Autodesk Inventor part; units mm, degrees
ref_plane "YZ Plane" through (0, 0, 0) normal (1, 0, 0) x (0, 1, 0)
ref_plane "XZ Plane" through (0, 0, 0) normal (0, 1, 0) x (-1, 0, 0)
ref_plane "XY Plane" through (0, 0, 0) normal (0, 0, 1) x (1, 0, 0)
sketch "Sketch1" plane through (0, 0, 0) normal (0, 1, 0) x (-1, 0, 0)
  circle A0 centre (0, 0) radius 39.5
  circle A1 centre (0, 0) radius 40.5
  dimension "d0" = 79
  dimension "d1" = 81
extrude "Extrusion1" add sketch "Sketch1" along normal blind 2
sketch "Sketch21" plane through (0, 2, 0) normal (0, 1, 0) x (1, 0, 0)
  line L0 (-40.5, -40.5) -> (40.5, -40.5)
  line L1 (40.5, -40.5) -> (40.5, 40.5)
  line L2 (40.5, 40.5) -> (-40.5, 40.5)
  line L3 (-40.5, 40.5) -> (-40.5, -40.5)
  line L4 (-40.5, -40.5) -> (40.5, 40.5) construction
  line L5 (40.5, -40.5) -> (-40.5, 40.5) construction
  circle A0 centre (0, 0) radius 40.5
  dimension "d111" = 81
  dimension "d112" = 81
extrude "Extrusion21" add sketch "Sketch21" against normal blind 2 contours L3 A0 L0 | A0 L1 L0 | L3 L2 A0 | A0 L2 L1
fillet "Fillet3" radius 20 4 edges at (-40.5, 1, -40.5) (40.5, 1, -40.5) (40.5, 1, 40.5) (-40.5, 1, 40.5)
sketch "Sketch24" plane through (0, 0, 0) normal (0, -1, 0) x (1, 0, 0)
  arc A0 (-20.5, 40.5) -> (-40.5, 20.5) centre (-20.5, 20.5) ccw
  circle A1 centre (0, 0) radius 39.5
  arc A2 (-20.5, 40.5) -> (-40.5, 20.5) centre (-20.5, 20.5) ccw
  line L0 (-40.5, 20.5) -> (-40.5, -20.5)
  arc A3 (-40.5, -20.5) -> (-20.5, -40.5) centre (-20.5, -20.5) ccw
  line L1 (-20.5, -40.5) -> (20.5, -40.5)
  arc A4 (20.5, -40.5) -> (40.5, -20.5) centre (20.5, -20.5) ccw
  line L2 (40.5, -20.5) -> (40.5, 20.5)
  arc A5 (40.5, 20.5) -> (20.5, 40.5) centre (20.5, 20.5) ccw
  line L3 (20.5, 40.5) -> (-20.5, 40.5)
  line L4 (-20, -40) -> (20, -40)
  line L5 (40, -20) -> (40, 20)
  line L6 (20, 40) -> (-20, 40)
  line L7 (-40, 20) -> (-40, -20)
  line L8 (-40, -40) -> (40, 40) construction
  line L9 (40, -40) -> (-40, 40) construction
  arc A6 (-38, 40) -> (-40, 38) centre (-38, 38) ccw
  arc A7 (40, 20) -> (20, 40) centre (20, 20) ccw
  arc A8 (-20, 40) -> (-40, 20) centre (-20, 20) ccw
  arc A9 (-40, -20) -> (-20, -40) centre (-20, -20) ccw
  arc A10 (20, -40) -> (40, -20) centre (20, -20) ccw
  dimension "d133" = 80
  dimension "d134" = 80
  dimension "d135" = 2
  dimension "d136" = 20
extrude "Extrusion24" add sketch "Sketch24" along normal blind 40 contours L3 A5 L2 A4 L1 A3 L0 A0
sketch "Sketch25" plane through (0, 0, 0) normal (0, -1, 0) x (1, 0, 0)
  circle A0 centre (-31, -31) radius 2
  line L0 (0, 0) -> (-40.0942, -40.0942)
  line L1 (0, 0) -> (0, -34.7078)
  circle A1 centre (31, -31) radius 2
  circle A2 centre (31, 31) radius 2
  circle A3 centre (-31, 31) radius 2
  dimension "d139" = 4
  dimension "d140" = 31
  dimension "d141" = 45
  dimension "d144" = 360
extrude "Extrusion25" cut sketch "Sketch25" against normal blind 10
properties part number "Motor mount (plain)"
Input: part model. Units: mm. Frame: model coordinates. A direction names the side the tool comes from. Give positions to 0.01 mm unless a question says otherwise; leave off trailing zeros. Order: outer loops, then holes, each group sorted by start corner. A loop starts at its lowest first (then second) coordinate and runs counter-clockwise, first axis right, second up. Notation, with made-up numbers: M 22.5,54 L 48.5,54 A26 cw 48.5,87 Z; hole C -24.5,-33.5 d1. An arc over 180 degrees is marked long. Return JSON: item names as keys, results as strings.
Item 1: Cut plane D-D (z = 31). Return loops of the section in (x, y), then the cut area to 3 significant figures.
Solutions:
{"outline": "M -37.52,-40 L -36.7,-40 L -36.7,0 L -33,0 L -33,2 L -37.52,2 Z; M -29,0 L -24.48,0 L -24.48,2 L -29,2 Z; M 24.48,0 L 29,0 L 29,2 L 24.48,2 Z; M 33,0 L 36.7,0 L 36.7,-40 L 37.52,-40 L 37.52,2 L 33,2 Z", "area": "102 mm^2"}
Item 2: Access query for faces 1 (the cylindrical face through (33.986, -19.72, 34.297)), 2 (the flat face through (0, -19, -40.5)). Directions: +Z, -Z, +X, -X, +Y, -Y. A direction counts if a zero-diameter tool reaches every point of the face in a straight line with its end or side. Return the directions, or none.
Solutions:
{"face 1": "-Y", "face 2": "-Z, +X, -X, +Y, -Y"}
Item 3: Ray query, probe 1 along Z at (x, y) = (-17.5, -27.5); probe 2 along Z at (x, y) = (31, 1). Return the intervals inside material, ascending.
Solutions:
{"probe 1": "-40.5 to -40, 40 to 40.5", "probe 2": "-37.52 to -33, -29 to -24.48, 24.48 to 29, 33 to 37.52"}
Item 4: First-contact query: P1, Ø8, axis at x = 18.5, z = -29.5, coming from the +Y side; P2, Ø5, axis at x = 31, z = 31, coming from the -Y side. Flat tips, straight axial feed; report the tip coordinate or a pass-through.
Solutions:
{"P1": "through", "P2": "y = 0"}
Item 5: Cut plane C-C (y = -14). Return loops of the section in (x, z).
Solutions:
{"outline": "M -40.5,-20.5 A20 ccw -20.5,-40.5 L 20.5,-40.5 A20 ccw 40.5,-20.5 L 40.5,20.5 A20 ccw 20.5,40.5 L -20.5,40.5 A20 ccw -40.5,20.5 Z; hole M -40,-20 A20 ccw -20,-40 L 20,-40 A20 ccw 40,-20 L 40,20 A20 ccw 20,40 L -20,40 A20 ccw -40,20 Z"}
Item 6: Cut plane B-B (z = 0). Return loops of the section in (x, y).
Solutions:
{"outline": "M -40.5,-40 L -40,-40 L -40,0 L -39.5,0 L -39.5,2 L -40.5,2 Z; M 39.5,0 L 40,0 L 40,-40 L 40.5,-40 L 40.5,2 L 39.5,2 Z"}
Item 7: Pull-direction query (Z, two-part tool) for faces 3 (the cylindrical face through (31.923, 0.986, 29.226)), 4 (the flat face through (40.5, -19, 0)), 5 (the flat face through (0, -20, 40)), 6 (the flat face through (0, -19, 40.5)); classes: +Z half, -Z half, draft (parallel to the pull), parting line (faces both ways), or undercut.
Solutions:
{"face 3": "undercut", "face 4": "draft", "face 5": "undercut", "face 6": "+Z half"}
Item 8: Cut plane A-A (x = 0). Return loops of the section in (y, z).
Solutions:
{"outline": "M -40,-40.5 L 2,-40.5 L 2,-39.5 L 0,-39.5 L 0,-40 L -40,-40 Z; M -40,40 L 0,40 L 0,39.5 L 2,39.5 L 2,40.5 L -40,40.5 Z"}
